The model under review builds one solid part; all positions refer to its coordinate system, in mm. A direction names the side the tool comes from. Give positions to 0.01 mm unless a question says otherwise; leave off trailing zeros. Order: outer loops, then holes, each group sorted by start corner. A loop starts at its lowest first (then second) coordinate and runs counter-clockwise, first axis right, second up. Notation, with made-up numbers: (20, 55.5) - (35, 55.5) arc R11 ccw to (35, 60.5) - close; hole circle Ø9 at (50, -1.75). An arc over 180 degrees is marked (long way). Use CSV: the item, a comma, the result in double quotes. Start each with the question number.
1. To check wall thickness, follow line 1 (Z direction, x = 6, y = 47); line 2 (Z direction, x = 7, y = 6); line 3 (Y direction, x = -21, z = -27). State the ranges of each line that lie inside material, in increasing order. Write a range as [from, to].
2. Machinability: for faces 4 (the cylindrical face through (7.79, 4.61, 26.78)), 5 (the flat face through (-48, 25, -28)), 6 (the flat face through (-61, 56, -10.176)), 7 (the flat face through (-57.715, 56, -13)), 8 (the flat face through (-7.715, 56, 35)), which of the approach directions +Z, -Z, +X, -X, +Y, -Y give a long, thin tool a straight path to every point of the face, cutting with its end or side? Answer none if there is none.
3. Draft analysis for pull direction Z (two halves, no side actions). For faces 1 (the flat face through (7.285, 45, -17)), 2 (the flat face through (-61, 56, -16.176)), 3 (the flat face through (3, 58.5, -13)), state which applies: released by +Z, released by -Z, zero draft, split by the parting line, or undercut.
4. Take a section at B-B, the plane x = -26. State the section outline as (y, z) points.
5. Take a section at D-D, the plane y = 27. State the section outline as (x, z) points, then the cut area to 3 significant figures.
6. For pin 1 (3.5 mm diameter, centred on y = 47.5, z = -16.68, fed in from -X); pin 2 (10 mm diameter, centred on y = -26.5, z = -2, fed in from +X); pin 3 (3.5 mm diameter, centred on y = 57, z = -12, fed in from -X); pin 4 (2.5 mm diameter, centred on x = -29, z = 3, fed in from -Y), all flat-tipped, find the tip position at first contact; note any pin that passes through.
7. Take a section at A-A, the plane y = -18. State the section outline as (x, z) points, then the cut area to 3 significant figures.
8. Take a section at C-C, the plane z = -9. State the section outline as (x, y) points.
```python
from build123d import *

# Parameters (mm, degrees)
SKETCH_1_W          = 74
SKETCH_1_H          = 72
EXTRUDE_1_DEPTH     = 54
SKETCH_2_W          = 70
SKETCH_2_H          = 68
CUT_EXTRUDE_1_DEPTH = 52
SKETCH_4_R          = 23.5
SKETCH_4_R_2        = 2
CUT_EXTRUDE_2_DEPTH = 2
SKETCH_5_W          = 14
SKETCH_5_H          = 68
CUT_EXTRUDE_3_DEPTH = 2
SKETCH_6_W          = 9
SKETCH_6_H          = 2
EXTRUDE_2_DEPTH     = 5
SKETCH_7_W          = 9
SKETCH_7_H          = 2
EXTRUDE_3_DEPTH     = 5
CUT_EXTRUDE_4_REACH = 101.89
SKETCH_9_W          = 64
SKETCH_9_H          = 46
SKETCH_10_W         = 4
SKETCH_10_H         = 8
EXTRUDE_5_DEPTH     = 5
SKETCH_11_W         = 4
SKETCH_11_H         = 8
EXTRUDE_6_DEPTH     = 5
SKETCH_15_W         = 70
SKETCH_15_H         = 68
EXTRUDE_7_DEPTH     = 2
SKETCH_16_W         = 6
SKETCH_16_H         = 6
EXTRUDE_8_DEPTH     = 4.5
SKETCH_17_W         = 2
SKETCH_17_H         = 2
EXTRUDE_9_DEPTH     = 1
SKETCH_18_W         = 2
SKETCH_18_H         = 2
EXTRUDE_10_DEPTH    = 1
SKETCH_19_W         = 2
SKETCH_19_H         = 2
EXTRUDE_11_DEPTH    = 1
SKETCH_20_W         = 2
SKETCH_20_H         = 2
EXTRUDE_12_DEPTH    = 1
CUT_EXTRUDE_5_REACH = 94.782
SKETCH_21_W         = 7.5
SKETCH_21_H         = 7.5
SKETCH_25_W         = 20
SKETCH_25_H         = 10
EXTRUDE_15_DEPTH    = 30
SKETCH_26_R         = 10
EXTRUDE_16_DEPTH    = 10
SKETCH_27_R         = 2
CUT_EXTRUDE_6_DEPTH = 10
CUT_EXTRUDE_7_REACH = 90.422
SKETCH_29_W         = 3
SKETCH_29_H         = 27
CUT_EXTRUDE_8_REACH = 106.96
SKETCH_30_W         = 3
SKETCH_30_H         = 3
CHAMFER_1_SIZE      = 1
CHAMFER_2_SIZE      = 1
SKETCH_31_R         = 3.1
CUT_EXTRUDE_9_DEPTH = 1
CHAMFER_3_SIZE      = 1


with BuildPart() as part:
    # 草图1 → 凸台-拉伸1 (new body)
    with BuildSketch(Plane(origin=(0, 0, 0), x_dir=(1, 0, 0), z_dir=(0, 1, 0))):
        with Locations((-28.715316709, -3.823796856)):
            Rectangle(SKETCH_1_W, SKETCH_1_H)
    extrude(amount=EXTRUDE_1_DEPTH)

    # 草图2 → 切除-拉伸1 (cut)
    with BuildSketch(Plane(origin=(0, 54, 0), x_dir=(1, 0, 0), z_dir=(0, 1, 0))):
        with Locations((-28.715316709, -3.823796856)):
            Rectangle(SKETCH_2_W, SKETCH_2_H)
    extrude(amount=-CUT_EXTRUDE_1_DEPTH, mode=Mode.SUBTRACT)

    # 草图4 → 切除-拉伸2 (cut)
    with BuildSketch(Plane(origin=(8.284683291, 0, 0), x_dir=(0, 0, -1), z_dir=(1, 0, 0))):
        with Locations((-3.823796856, 27)):
            Circle(SKETCH_4_R)
        with Locations((16.676203144, 6.5)):
            Circle(SKETCH_4_R_2)
        with Locations((-24.323796856, 47.5)):
            Circle(SKETCH_4_R_2)
        with Locations((-24.323796856, 6.5)):
            Circle(SKETCH_4_R_2)
        with Locations((16.676203144, 47.5)):
            Circle(SKETCH_4_R_2)
    extrude(amount=-CUT_EXTRUDE_2_DEPTH, mode=Mode.SUBTRACT)

    # 草图5 → 切除-拉伸3 (cut)
    with BuildSketch(Plane.XZ):
        with Locations((-56.715316709, 3.823796856)):
            Rectangle(SKETCH_5_W, SKETCH_5_H)
    extrude(amount=-CUT_EXTRUDE_3_DEPTH, mode=Mode.SUBTRACT)

    # 草图6 → 凸台-拉伸2 (add)
    with BuildSketch(Plane(origin=(0, 0, 37.823796856), x_dir=(-1, 0, 0), z_dir=(0, 0, -1))):
        with Locations((59.215316709, 53)):
            Rectangle(SKETCH_6_W, SKETCH_6_H)
    extrude(amount=EXTRUDE_2_DEPTH)

    # 草图7 → 凸台-拉伸3 (add)
    with BuildSketch(Plane.XY.offset(-30.176203144)):
        with Locations((-59.215316709, 53)):
            Rectangle(SKETCH_7_W, SKETCH_7_H)
    extrude(amount=EXTRUDE_3_DEPTH)

    # 草图9 → 切除-拉伸4 (cut, up to next)
    with BuildSketch(Plane.ZY.offset(65.715316709), mode=Mode.PRIVATE) as cut_extrude_4_sk1:
        with Locations((3.823796856, 27)):
            Rectangle(SKETCH_9_W, SKETCH_9_H)
    cut_extrude_4_tool1 = extrude(cut_extrude_4_sk1.sketch, amount=-CUT_EXTRUDE_4_REACH, mode=Mode.PRIVATE) & part.part
    add(cut_extrude_4_tool1.solids().sort_by_distance((-65.715317, 27, 3.823797))[0], mode=Mode.SUBTRACT)

    # 草图10 → 凸台-拉伸5 (add)
    with BuildSketch(Plane(origin=(0, 0, 37.823796856), x_dir=(-1, 0, 0), z_dir=(0, 0, -1))):
        with Locations((47.715316709, 14)):
            Rectangle(SKETCH_10_W, SKETCH_10_H)
        with Locations((47.715316709, 29)):
            Rectangle(SKETCH_10_W, SKETCH_10_H)
        with Locations((47.715316709, 44)):
            Rectangle(SKETCH_10_W, SKETCH_10_H)
    extrude(amount=EXTRUDE_5_DEPTH)

    # 草图11 → 凸台-拉伸6 (add)
    with BuildSketch(Plane.XY.offset(-30.176203144)):
        with Locations((-47.715316709, 14)):
            Rectangle(SKETCH_11_W, SKETCH_11_H)
        with Locations((-47.715316709, 29)):
            Rectangle(SKETCH_11_W, SKETCH_11_H)
        with Locations((-47.715316709, 44)):
            Rectangle(SKETCH_11_W, SKETCH_11_H)
    extrude(amount=EXTRUDE_6_DEPTH)

    # 草图15 → 凸台-拉伸7 (add)
    with BuildSketch(Plane(origin=(0, 54, 0), x_dir=(1, 0, 0), z_dir=(0, 1, 0))):
        with Locations((-28.715316709, -3.823796856)):
            Rectangle(SKETCH_15_W, SKETCH_15_H)
    extrude(amount=-EXTRUDE_7_DEPTH)

    # 草图16 → 凸台-拉伸8 (add)
    with BuildSketch(Plane(origin=(0, 54, 0), x_dir=(1, 0, 0), z_dir=(0, 1, 0))):
        with Locations((-46.715316709, -34.823796856)):
            Rectangle(SKETCH_16_W, SKETCH_16_H)
        with Locations((-60.715316709, 13.176203144)):
            Rectangle(SKETCH_16_W, SKETCH_16_H)
        with Locations((-10.715316709, -34.823796856)):
            Rectangle(SKETCH_16_W, SKETCH_16_H)
        with Locations((-46.715316709, 27.176203144)):
            Rectangle(SKETCH_16_W, SKETCH_16_H)
        with Locations((-10.715316709, 27.176203144)):
            Rectangle(SKETCH_16_W, SKETCH_16_H)
        with Locations((3.284683291, 13.176203144)):
            Rectangle(SKETCH_16_W, SKETCH_16_H)
        with Locations((3.284683291, -20.823796856)):
            Rectangle(SKETCH_16_W, SKETCH_16_H)
        with Locations((-60.715316709, -20.823796856)):
            Rectangle(SKETCH_16_W, SKETCH_16_H)
    extrude(amount=EXTRUDE_8_DEPTH)

    # 草图17 → 凸台-拉伸9 (add)
    with BuildSketch(Plane.ZY.offset(63.715316709)):
        with Locations((-13.176203144, 57)):
            Rectangle(SKETCH_17_W, SKETCH_17_H)
        with Locations((20.823796856, 57)):
            Rectangle(SKETCH_17_W, SKETCH_17_H)
    extrude(amount=EXTRUDE_9_DEPTH)

    # 草图18 → 凸台-拉伸10 (add)
    with BuildSketch(Plane.XY.offset(37.823796856)):
        with Locations((-10.715316709, 57)):
            Rectangle(SKETCH_18_W, SKETCH_18_H)
        with Locations((-46.715316709, 57)):
            Rectangle(SKETCH_18_W, SKETCH_18_H)
    extrude(amount=EXTRUDE_10_DEPTH)

    # 草图19 → 凸台-拉伸11 (add)
    with BuildSketch(Plane(origin=(6.284683291, 0, 0), x_dir=(0, 0, -1), z_dir=(1, 0, 0))):
        with Locations((13.176203144, 57)):
            Rectangle(SKETCH_19_W, SKETCH_19_H)
        with Locations((-20.823796856, 57)):
            Rectangle(SKETCH_19_W, SKETCH_19_H)
    extrude(amount=EXTRUDE_11_DEPTH)

    # 草图20 → 凸台-拉伸12 (add)
    with BuildSketch(Plane(origin=(0, 0, -30.176203144), x_dir=(-1, 0, 0), z_dir=(0, 0, -1))):
        with Locations((46.715316709, 57)):
            Rectangle(SKETCH_20_W, SKETCH_20_H)
        with Locations((10.715316709, 57)):
            Rectangle(SKETCH_20_W, SKETCH_20_H)
    extrude(amount=EXTRUDE_12_DEPTH)

    # 草图21 → 切除-拉伸5 (cut, up to next)
    with BuildSketch(Plane(origin=(0, 52, 0), x_dir=(-1, 0, 0), z_dir=(0, -1, 0)), mode=Mode.PRIVATE) as cut_extrude_5_sk1:
        with Locations((13.936875607, -11.824892758)):
            Rectangle(SKETCH_21_W, SKETCH_21_H)
    cut_extrude_5_tool1 = extrude(cut_extrude_5_sk1.sketch, amount=-CUT_EXTRUDE_5_REACH, mode=Mode.PRIVATE) & part.part
    # 草图21 → 切除-拉伸5 (cut, up to next)
    with BuildSketch(Plane(origin=(0, 52, 0), x_dir=(-1, 0, 0), z_dir=(0, -1, 0)), mode=Mode.PRIVATE) as cut_extrude_5_sk2:
        with Locations((13.936875607, 7.433232356)):
            Rectangle(SKETCH_21_W, SKETCH_21_H)
    cut_extrude_5_tool2 = extrude(cut_extrude_5_sk2.sketch, amount=-CUT_EXTRUDE_5_REACH, mode=Mode.PRIVATE) & part.part
    add(cut_extrude_5_tool1.solids().sort_by_distance((-13.936876, 52, 11.824893))[0], mode=Mode.SUBTRACT)
    add(cut_extrude_5_tool2.solids().sort_by_distance((-13.936876, 52, -7.433232))[0], mode=Mode.SUBTRACT)

    # 草图25 → 凸台-拉伸15 (add)
    with BuildSketch(Plane.XZ):
        with Locations((-34.727823945, 3.823796856)):
            Rectangle(SKETCH_25_W, SKETCH_25_H)
    extrude(amount=EXTRUDE_15_DEPTH)

    # 草图26 → 凸台-拉伸16 (add)
    with BuildSketch(Plane.XY.offset(8.823796856)):
        with Locations((-34.727823945, -30)):
            Circle(SKETCH_26_R)
    extrude(amount=-EXTRUDE_16_DEPTH)

    # 草图27 → 切除-拉伸6 (cut)
    with BuildSketch(Plane.XY.offset(8.823796856)):
        with Locations((-34.727823945, -30)):
            Circle(SKETCH_27_R)
    extrude(amount=-CUT_EXTRUDE_6_DEPTH, mode=Mode.SUBTRACT)

    # 草图29 → 切除-拉伸7 (cut, up to next)
    with BuildSketch(Plane.ZY.offset(44.727823945), mode=Mode.PRIVATE) as cut_extrude_7_sk1:
        with Locations((3.823796856, -26.5)):
            Rectangle(SKETCH_29_W, SKETCH_29_H)
    cut_extrude_7_tool1 = extrude(cut_extrude_7_sk1.sketch, amount=-CUT_EXTRUDE_7_REACH, mode=Mode.PRIVATE) & part.part
    add(cut_extrude_7_tool1.solids().sort_by_distance((-44.727824, -26.5, 3.823797))[0], mode=Mode.SUBTRACT)

    # 草图30 → 切除-拉伸8 (cut, up to next)
    with BuildSketch(Plane.XZ.offset(13), mode=Mode.PRIVATE) as cut_extrude_8_sk1:
        with Locations((-34.727823945, 3.823796856)):
            Rectangle(SKETCH_30_W, SKETCH_30_H)
    cut_extrude_8_tool1 = extrude(cut_extrude_8_sk1.sketch, amount=-CUT_EXTRUDE_8_REACH, mode=Mode.PRIVATE) & part.part
    add(cut_extrude_8_tool1.solids().sort_by_distance((-34.727824, -13, 3.823797))[0], mode=Mode.SUBTRACT)

    # 倒角1
    chamfer_1_edges = [part.edges().sort_by_distance(p)[0] for p in [
        (-28.715316709, 0, -32.176203144),
        (8.284683291, 0, 3.823796856),
        (-28.715316709, 0, 39.823796856),
        (-65.715316709, 0, 3.823796856),
        (-65.715316709, 27, -32.176203144),
        (8.284683291, 27, -32.176203144),
        (8.284683291, 27, 39.823796856),
        (-65.715316709, 27, 39.823796856),
    ]]
    chamfer(chamfer_1_edges, length=CHAMFER_1_SIZE)

    # 倒角2
    chamfer_2_edges = [part.edges().sort_by_distance(p)[0] for p in [
        (7.284683291, 58, 20.823796856),
        (7.284683291, 58, -13.176203144),
        (-10.715316709, 58, -31.176203144),
        (-46.715316709, 58, -31.176203144),
        (-64.715316709, 58, -13.176203144),
        (-64.715316709, 58, 20.823796856),
        (-10.715316709, 58, 38.823796856),
        (-46.715316709, 58, 38.823796856),
    ]]
    chamfer(chamfer_2_edges, length=CHAMFER_2_SIZE - 0.0001)  # a hair under: the kernel refuses the full size

    # 草图31 → 切除-拉伸9 (cut)
    with BuildSketch(Plane(origin=(8.284683291, 0, 0), x_dir=(0, 0, -1), z_dir=(1, 0, 0))):
        with Locations((16.676203144, 6.5)):
            Circle(SKETCH_31_R)
        with Locations((-24.323796856, 6.5)):
            Circle(SKETCH_31_R)
        with Locations((-24.323796856, 47.5)):
            Circle(SKETCH_31_R)
        with Locations((16.676203144, 47.5)):
            Circle(SKETCH_31_R)
    extrude(amount=-CUT_EXTRUDE_9_DEPTH, mode=Mode.SUBTRACT)

    # 倒角3
    chamfer_3_edges = [part.edges().sort_by_distance(p)[0] for p in [
        (-64.715316709, 56, 20.823796856),
        (-64.715316709, 56, -13.176203144),
        (-46.715316709, 56, -31.176203144),
        (-10.715316709, 56, -31.176203144),
        (7.284683291, 56, -13.176203144),
        (7.284683291, 56, 20.823796856),
        (-46.715316709, 56, 38.823796856),
        (-10.715316709, 56, 38.823796856),
    ]]
    chamfer(chamfer_3_edges, length=CHAMFER_3_SIZE - 0.0001)  # a hair under: the kernel refuses the full size


solid = part.part
```
Determined:
1,line 1,"z = [-32.18, -30.18], [37.82, 39.82]"
1,line 2,"z = [-32.18, -18.61], [-14.74, -6.72], [14.37, 22.39], [26.26, 39.82]"
1,line 3,"y = [0, 2], [52, 54]"
2,face 4,"+X"
2,face 5,"none"
2,face 6,"+X, -X, +Y"
2,face 7,"+Z, -Z, +Y"
2,face 8,"+Z, -Z, +X, +Y"
3,face 1,"undercut"
3,face 2,"released by -Z"
3,face 3,"zero draft"
4,outline,"(-34.88, -1.18) - (0, -1.18) - (0, -31.18) - (1, -32.18) - (54, -32.18) - (54, 39.82) - (1, 39.82) - (0, 38.82) - (0, 8.82) - (-34.88, 8.82) - (-34.88, 5.32) - (-13, 5.32) - (-13, 2.32) - (-34.88, 2.32) - close; hole (2, -30.18) - (52, -30.18) - (52, 37.82) - (2, 37.82) - close"
5,outline,"(-65.72, -31.18) - (-64.72, -32.18) - (7.28, -32.18) - (8.28, -31.18) - (8.28, -19.68) - (6.28, -19.68) - (6.28, -30.18) - (-45.72, -30.18) - (-45.72, -25.18) - (-49.72, -25.18) - (-49.72, -30.18) - (-63.72, -30.18) - (-63.72, -28.18) - (-65.72, -28.18) - close; (-65.72, 35.82) - (-63.72, 35.82) - (-63.72, 37.82) - (-49.72, 37.82) - (-49.72, 32.82) - (-45.72, 32.82) - (-45.72, 37.82) - (6.28, 37.82) - (6.28, 27.32) - (8.28, 27.32) - (8.28, 38.82) - (7.28, 39.82) - (-64.72, 39.82) - (-65.72, 38.82) - close"
5,area,"384 mm²"
6,pin 1,"passes through"
6,pin 2,"stops at x = -24.73"
6,pin 3,"stops at x = -64.72"
6,pin 4,"stops at y = -38.84"
7,outline,"(-44.73, -1.18) - (-24.73, -1.18) - (-24.73, 2.32) - (-44.73, 2.32) - close; (-44.73, 5.32) - (-24.73, 5.32) - (-24.73, 8.82) - (-44.73, 8.82) - close"
7,area,"140 mm²"
8,outline,"(-65.72, 1) - (-64.72, 0) - (-63.72, 0) - (-63.72, 4) - (-65.72, 4) - close; (-65.72, 50) - (-63.72, 50) - (-63.72, 52) - (-17.69, 52) - (-17.69, 54) - (-65.72, 54) - close; (-49.72, 0) - (7.28, 0) - (8.28, 1) - (8.28, 7.31) - (6.28, 7.31) - (6.28, 2) - (-49.72, 2) - close; (-10.19, 52) - (6.28, 52) - (6.28, 46.69) - (8.28, 46.69) - (8.28, 54) - (-10.19, 54) - close"
